```python
from build123d import *

# Parameters (mm, degrees)
SKETCH1_R           = 17.5
BOSS_EXTRUDE1_DEPTH = 23
SKETCH2_R           = 17
BOSS_EXTRUDE2_DEPTH = 50
SKETCH3_R           = 5
BOSS_EXTRUDE3_DEPTH = 2
BOSS_EXTRUDE4_DEPTH = 10


with BuildPart() as part:
    # Sketch1 → Boss-Extrude1 (new body)
    with BuildSketch(Plane.XY):
        Circle(SKETCH1_R)
    extrude(amount=BOSS_EXTRUDE1_DEPTH)

    # Sketch2 → Boss-Extrude2 (add)
    with BuildSketch(Plane.XY.offset(23)):
        Circle(SKETCH2_R)
    extrude(amount=BOSS_EXTRUDE2_DEPTH)

    # Sketch3 → Boss-Extrude3 (add)
    with BuildSketch(Plane(origin=(0, 0, 0), x_dir=(-1, 0, 0), z_dir=(0, 0, -1))):
        Circle(SKETCH3_R)
    extrude(amount=BOSS_EXTRUDE3_DEPTH)

    # Sketch4 → Boss-Extrude4 (add)
    with BuildSketch(Plane(origin=(0, 0, -2), x_dir=(-1, 0, 0), z_dir=(0, 0, -1))):
        with BuildLine():
            Line((2, 1.5), (-2, 1.5))
            ThreePointArc((-2, 1.5), (-0.790569415, -2.371708245), (2.5, 0))
            ThreePointArc((2.5, 0), (2.371708245, 0.790569415), (2, 1.5))
        make_face()
    extrude(amount=BOSS_EXTRUDE4_DEPTH)


solid = part.part
```
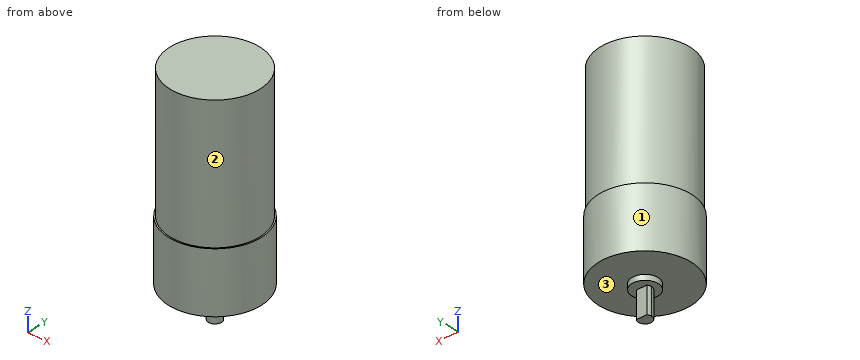
Source: CAD feature listing. Evaluate the final solid. Frame: model axes, mm. Face numbers are marked on the shaded views. A direction names the side the tool comes from. Round coordinates to 2 decimals unless told otherwise and drop trailing zeros. Loops run counter-clockwise (first coordinate to the right, second up) from the corner with the lowest first, then second, coordinate; pieces in that order, holes last. Notation, with made-up numbers: M -28,63.25 L 20,63.25 A18 ccw 20,90.25 Z; hole C 2,34.25 d4. An arc over 180 degrees is marked long. Put each result on its own line as item: value.
(1) Ray query, line 1 (Y direction, x = 0, z = -8); line 2 (Z direction, x = 11.5, y = 2.5); line 3 (Z direction, x = 13.5, y = -11). Return the intervals inside material, ascending. Write a range as [from, to].
Solutions:
line 1: [-2.5, 1.5]
line 2: [0, 73]
line 3: [0, 23]
(2) Section C-C, the plane z = 61. Return loops of the section in (x, y), and give its area (3 significant figures).
Solutions:
outline: C 0,0 d34
area: 908 mm²
(3) Section A-A, the plane x = 0. Return loops of the section in (y, z).
Solutions:
outline: M -17.5,0 L -5,0 L -5,-2 L -2.5,-2 L -2.5,-12 L 1.5,-12 L 1.5,-2 L 5,-2 L 5,0 L 17.5,0 L 17.5,23 L 17,23 L 17,73 L -17,73 L -17,23 L -17.5,23 Z
(4) Access query for the marked faces 1, 2 and 3. Directions: +Z, -Z, +X, -X, +Y, -Y. A direction counts if a zero-diameter tool reaches every point of the face in a straight line with its end or side. Return the directions, or none.
Solutions:
face 1: +Z, -Z
face 2: +Z
face 3: -Z
(5) Section D-D, the plane x = 6. Return loops of the section in (y, z), and give its area (3 significant figures).
Solutions:
outline: M -16.44,0 L 16.44,0 L 16.44,23 L 15.91,23 L 15.91,73 L -15.91,73 L -15.91,23 L -16.44,23 Z
area: 2,350 mm²
(6) Section B-B, the plane y = -14. Return loops of the section in (x, z), and give its area (3 significant figures).
Solutions:
outline: M -10.5,0 L 10.5,0 L 10.5,23 L 9.64,23 L 9.64,73 L -9.64,73 L -9.64,23 L -10.5,23 Z
area: 1,450 mm²
(7) First-contact query: pin 1 (3 mm diameter, centred on y = 0, z = 52.5, fed in from -X); pin 2 (1 mm diameter, centred on x = 11, y = -9.5, fed in from -Z); pin 3 (8 mm diameter, centred on x = 5.5, z = 8, fed in from -Y). Flat tips, straight axial feed; report the tip coordinate or a pass-through.
Solutions:
pin 1: x = -17
pin 2: z = 0
pin 3: y = -17.44
